Verification items for the finished model (mm, model axes). A direction names the side the tool comes from. Coordinates: 2 decimals unless noted, no trailing zeros. Write each loop counter-clockwise with the first axis right and the second up, starting at its lowest first coordinate (ties: lowest second). Pieces come first, ordered by that corner, then holes. Notation, with made-up numbers: (46.5, 74) -> (79.5, 74) arc R9 ccw to (79.5, 85) -> close; hole circle Ø9 at (61.5, 27). An arc over 180 degrees is marked (long way). Write each question's results on one line, items separated by ' | '. Start each with the question number.
from build123d import *

# Parameters (mm, degrees)
F0_W     = 50.8
F0_H     = 34.935082
F0_R     = 9.525
F1_DEPTH = 2.54
F0_H_2   = 3.164918
F2_DEPTH = 25.4
F3_R     = 5.08
F4_R     = 3.175
F5_DEPTH = 25.4


with BuildPart() as f1:
    # F0 (on Front) → F1 (new body)
    with BuildSketch(Plane.XZ):
        with Locations((-7.487633, -19.108459)):
            Rectangle(F0_W, F0_H)
        with Locations((-7.487633, -23.876)):
            Circle(F0_R, mode=Mode.SUBTRACT)
    extrude(amount=F1_DEPTH)

    # F0 (on Front) → F2 (join)
    with BuildSketch(Plane.XZ):
        with Locations((-7.487633, -0.058459)):
            Rectangle(F0_W, F0_H_2)
    extrude(amount=F2_DEPTH)

    # F3
    f3_edges = [f1.edges().sort_by_distance(p)[0] for p in [
        (-7.487633, -2.54, -1.640918),
        (-7.487633, 0, 1.524),
    ]]
    fillet(f3_edges, radius=F3_R)

    # F4 (on face) → F5 (cut)
    with BuildSketch(Plane(origin=(0, 0, -1.640918), x_dir=(1, 0, 0), z_dir=(0, 0, -1))):
        with Locations((-20.187633, 16.51)):
            Circle(F4_R)
        with Locations((5.212367, 16.51)):
            Circle(F4_R)
    extrude(amount=-F5_DEPTH, mode=Mode.SUBTRACT)


solid = f1.part
1. Sectioned sample at C-C on z = -28. Record the cut outline in (x, y).
2. Mould release check, pull along Y, two halves, no side actions. Record for faces 1 (the cylindrical face through (2.04, -16.65, -0.08)), 2 (the cylindrical face through (-7.13, -1.45, 0)), 3 (the flat face through (-32.888, -2, -12)): +Y half, -Y half, draft (parallel to the pull), parting line (faces both ways), or undercut.
3. Sectioned sample at D-D on y = -10. Record the cut outline in (x, z), plus the area to 3 significant figures.
4. Sectioned sample at B-B on x = -4.5. Record the cut outline in (y, z), plus the area to 3 significant figures.
5. Depth check by flat-ended pin: pin 1 Ø5.5 at (x, y) = (-20.19, -16.51) entering from +Z (3 decimals); pin 2 Ø3 at (x, z) = (8.5, -7.5) entering from -Y; pin 3 Ø5.5 at (x, y) = (-10.5, -14) entering from -Z. Enter the tip coordinate at first touch or a pass-through.
6. Material ranges on probe 1 along X at (y, z) = (-16.51, -0.2); probe 2 along Z at (x, y) = (-7, -14.25); probe 3 along Y at (x, z) = (-0.5, -33.5), recorded low to high. Write a range as from..to.
7. Sectioned sample at A-A on y = -16.51. Record the cut outline in (x, z).
8. Tool access check on faces 4 (the flat face through (-8, -1, -36.576)), 5 (the flat face through (-13, -2.54, -15)). Record the directions out of +Z, -Z, +X, -X, +Y, -Y that give a thin tool (end or side, any length) a straight path to the whole face; none if there is none.
Computed values:
1) outline: (-32.89, -2.54) -> (-16.07, -2.54) -> (-16.07, 0) -> (-32.89, 0) -> close; (1.1, -2.54) -> (17.91, -2.54) -> (17.91, 0) -> (1.1, 0) -> close
2) face 1: undercut | face 2: +Y half | face 3: draft
3) outline: (-32.89, -1.64) -> (17.91, -1.64) -> (17.91, 1.52) -> (-32.89, 1.52) -> close | area: 161 mm^2
4) outline: (-25.4, -1.64) -> (-7.62, -1.64) arc R5.08 cw to (-2.54, -6.72) -> (-2.54, -14.83) -> (0, -14.83) -> (0, -3.56) arc R5.08 ccw to (-5.08, 1.52) -> (-25.4, 1.52) -> close; (-2.54, -36.58) -> (0, -36.58) -> (0, -32.92) -> (-2.54, -32.92) -> close | area: 123 mm^2
5) pin 1: passes through | pin 2: stops at y = -2.59 | pin 3: stops at z = -1.64
6) probe 1: x = -32.89..-23.36, -17.01..2.04, 8.39..17.91 | probe 2: z = -1.64..1.52 | probe 3: y = -2.54..0
7) outline: (-32.89, -1.64) -> (-23.36, -1.64) -> (-23.36, 1.52) -> (-32.89, 1.52) -> close; (-17.01, -1.64) -> (2.04, -1.64) -> (2.04, 1.52) -> (-17.01, 1.52) -> close; (8.39, -1.64) -> (17.91, -1.64) -> (17.91, 1.52) -> (8.39, 1.52) -> close
8) face 4: -Z, +X, -X, +Y, -Y | face 5: -Z, +X, -X, -Y
